Work out the finished part from the listing and answer in its coordinate system (mm). A direction names the side the tool comes from. Coordinates: 2 decimals unless noted, no trailing zeros. Write each loop counter-clockwise with the first axis right and the second up, starting at its lowest first coordinate (ties: lowest second). Pieces come first, ordered by that corner, then holes. Notation, with made-up numbers: (37.5, 60) - (87.5, 60) arc R18 cw to (87.5, 86) - close; hole circle Ø7 at (35.25, 24.25). An arc over 180 degrees is marked (long way). Use CSV: the item, a comma, the result in double quotes. Start each with the question number.
from build123d import *

# Parameters (mm, degrees)
EXTRUDE_1_DEPTH = 10
FILLET_1_R      = 5


with BuildPart() as part:
    # 草图1 → 凸台-拉伸1 (new body)
    with BuildSketch(Plane.XY):
        with BuildLine():
            Line((0, -1.5), (-30, -1.5))
            Line((-30, -1.5), (-35, -1.5))
            Line((-35, -1.5), (-35, 14.176056338))
            Line((-35, 14.176056338), (-30, 14.176056338))
            Line((-30, 14.176056338), (-30, 6.5))
            ThreePointArc((-30, 6.5), (-28.535533906, 2.964466094), (-25, 1.5))
            Line((-25, 1.5), (0, 1.5))
            ThreePointArc((0, 1.5), (1.5, 0), (0, -1.5))
        make_face()
    extrude(amount=EXTRUDE_1_DEPTH)

    # 圆角1
    fillet_1_edges = [part.edges().sort_by_distance(p)[0] for p in [
        (-35, -1.5, 5),
    ]]
    fillet(fillet_1_edges, radius=FILLET_1_R)


solid = part.part
Item 1: Which of the six approach directions +Z, -Z, +X, -X, +Y, -Y give full straight-line access (tool end or side, diameter ignored) to faces 1 (the face through (-21, 1, 10)), 2 (the face through (-13, 1.5, 5))?
Item 2: Each of these flat-tipped pins is pushed along its axis until it touches: pin 1 (3 mm diameter, centred on y = 4, z = 9, fed in from +X); pin 2 (1.5 mm diameter, centred on x = -14.5, y = 1, fed in from -Z); pin 3 (3 mm diameter, centred on x = -8, z = 4.5, fed in from +Y); pin 4 (6 mm diameter, centred on y = 10.5, z = 4, fed in from +X). Where does it stop, or does it pass through?
Item 3: A cutting plane is placed at C-C (y = 4). Determine the outline of the cut face in (x, z), then the cut area to 3 significant figures.
Item 4: A cutting plane is placed at A-A (z = 7.25). Determine the outline of the cut face in (x, y).
Item 5: A cutting plane is placed at B-B (x = -21). Determine the outline of the cut face in (y, z).
Item 6: Straight lines are drawn through the part: probe 1 along Y at (x, z) = (-16.5, 8.5); probe 2 along X at (y, z) = (9.5, 4.75); probe 3 along Y at (x, z) = (-29, 0.5). For each, find the intervals that lie inside material, in ascending order. Write a range as [from, to].
Calculated:
1,face 1,"+Z, +X, -X, +Y, -Y"
1,face 2,"+Z, -Z, +X, +Y"
2,pin 1,"stops at x = -28"
2,pin 2,"stops at z = 0"
2,pin 3,"stops at y = 1.5"
2,pin 4,"stops at x = -30"
3,outline,"(-35, 0) - (-29.33, 0) - (-29.33, 10) - (-35, 10) - close"
3,area,"56.7 mm²"
4,outline,"(-35, 3.5) arc R5 ccw to (-30, -1.5) - (0, -1.5) arc R1.5 ccw to (0, 1.5) - (-25, 1.5) arc R5 cw to (-30, 6.5) - (-30, 14.18) - (-35, 14.18) - close"
5,outline,"(-1.5, 0) - (1.5, 0) - (1.5, 10) - (-1.5, 10) - close"
6,probe 1,"y = [-1.5, 1.5]"
6,probe 2,"x = [-35, -30]"
6,probe 3,"y = [-1.5, 3.5]"
